```python
from build123d import *

# Parameters (mm, degrees)
CROQUIS1_W                  = 248.76
CROQUIS1_H                  = 195
SALIENTE_EXTRUIR1_DEPTH     = 5
CROQUIS2_W                  = 48
CROQUIS2_H                  = 30
CROQUIS2_W_2                = 30
CORTAR_EXTRUIR1_DEPTH       = 2
CROQUIS3_R                  = 2.375
CORTAR_EXTRUIR2_DEPTH       = 10
CROQUIS4_R                  = 40
SALIENTE_EXTRUIR2_DEPTH     = 206
CROQUIS5_R                  = 12.5
CORTAR_EXTRUIR3_DEPTH       = 10
CROQUIS12_W                 = 12
CROQUIS12_H                 = 30
SALIENTE_EXTRUIR3_DEPTH     = 4
REDONDEO1_R                 = 10
REDONDEO2_R                 = 10
REDONDEO3_R                 = 10
CORTAR_EXTRUIR5_DEPTH       = 262.677217236
CORTAR_EXTRUIR5_DEPTH_BACK  = 262.677217236
CROQUIS13_R                 = 1.625
CORTAR_EXTRUIR7_DEPTH       = 2
CROQUIS16_R                 = 1.75
CORTAR_EXTRUIR9_DEPTH       = 20
CROQUIS17_W                 = 120.38
CROQUIS17_H                 = 213.212791717
CORTAR_EXTRUIR10_DEPTH      = 222
CORTAR_EXTRUIR14_DEPTH      = 165.272498417
CORTAR_EXTRUIR14_DEPTH_BACK = 165.272498417
CROQUIS18_W                 = 124.38
CROQUIS18_H                 = 195


with BuildPart() as part:
    # Croquis1 → Saliente-Extruir1 (new body)
    with BuildSketch(Plane.XY):
        with Locations((7.088293187, 0.26268)):
            Rectangle(CROQUIS1_W, CROQUIS1_H)
    extrude(amount=SALIENTE_EXTRUIR1_DEPTH)

    # Croquis2 → Cortar-Extruir1 (cut)
    with BuildSketch(Plane.XY.offset(5)):
        with Locations((-93.291706813, -82.23732)):
            Rectangle(CROQUIS2_W, CROQUIS2_H)
        with Locations((116.468293187, 82.76268)):
            Rectangle(CROQUIS2_W_2, CROQUIS2_H)
        with Locations((116.468293187, -82.23732)):
            Rectangle(CROQUIS2_W_2, CROQUIS2_H)
        with Locations((-93.291706813, 82.76268)):
            Rectangle(CROQUIS2_W, CROQUIS2_H)
    extrude(amount=-CORTAR_EXTRUIR1_DEPTH, mode=Mode.SUBTRACT)

    # Croquis3 → Cortar-Extruir2 (cut)
    with BuildSketch(Plane.XY.offset(5)):
        with Locations((-93.291706813, 83.76268)):
            Circle(CROQUIS3_R)
        with Locations((-93.291706813, -83.23732)):
            Circle(CROQUIS3_R)
        with Locations((116.468293187, 83.76268)):
            Circle(CROQUIS3_R)
        with Locations((116.468293187, -83.23732)):
            Circle(CROQUIS3_R)
    extrude(amount=-CORTAR_EXTRUIR2_DEPTH, mode=Mode.SUBTRACT)

    # Croquis4 → Saliente-Extruir2 (add)
    with BuildSketch(Plane(origin=(0, 0, 0), x_dir=(-1, 0, 0), z_dir=(0, 0, -1))):
        with Locations(Location((55.101706813, 0.26268, 0), (0, 0, 180))):
            Circle(CROQUIS4_R)
    extrude(amount=SALIENTE_EXTRUIR2_DEPTH)

    # Croquis5 → Cortar-Extruir3 (cut)
    with BuildSketch(Plane(origin=(0, 0, 0), x_dir=(-1, 0, 0), z_dir=(0, 0, -1))):
        with Locations((-76.968293187, 0.26268)):
            Circle(CROQUIS5_R)
    extrude(amount=-CORTAR_EXTRUIR3_DEPTH, mode=Mode.SUBTRACT)

    # Croquis12 → Saliente-Extruir3 (add, symmetric)
    with BuildSketch(Plane(origin=(7.088293187, 0, 0), x_dir=(0, 0, -1), z_dir=(1, 0, 0))):
        with Locations((6, 82.76268)):
            Rectangle(CROQUIS12_W, CROQUIS12_H)
        with Locations((6, -82.23732)):
            Rectangle(CROQUIS12_W, CROQUIS12_H)
    extrude(amount=SALIENTE_EXTRUIR3_DEPTH, both=True)

    # Redondeo1
    redondeo1_edges = [part.edges().sort_by_distance(p)[0] for p in [
        (7.088293187, 67.76268, 0),
        (7.088293187, -67.23732, 0),
    ]]
    fillet(redondeo1_edges, radius=REDONDEO1_R)

    # Redondeo2
    redondeo2_edges = [part.edges().sort_by_distance(p)[0] for p in [
        (7.088293187, 67.76268, -12),
        (7.088293187, -67.23732, -12),
    ]]
    fillet(redondeo2_edges, radius=REDONDEO2_R)

    # Redondeo3
    redondeo3_edges = [part.edges().sort_by_distance(p)[0] for p in [
        (7.088293187, 97.76268, -12),
        (7.088293187, -97.23732, -12),
    ]]
    fillet(redondeo3_edges, radius=REDONDEO3_R)

    # Croquis13 → Cortar-Extruir5 (cut, two sides: drawn at the far end of the back side and taken through both)
    with BuildSketch(Plane(origin=(11.088293187, 0, 0), x_dir=(0, 0, -1), z_dir=(1, 0, 0)).offset(-CORTAR_EXTRUIR5_DEPTH_BACK)):
        with Locations(Location((6, 87.76268, 0), (0, 0, 90))):
            Circle(CROQUIS13_R)
        with Locations(Location((6, 77.76268, 0), (0, 0, 90))):
            Circle(CROQUIS13_R)
        with Locations(Location((6, -77.23732, 0), (0, 0, 90))):
            Circle(CROQUIS13_R)
        with Locations(Location((6, -87.23732, 0), (0, 0, 90))):
            Circle(CROQUIS13_R)
    extrude(amount=CORTAR_EXTRUIR5_DEPTH + CORTAR_EXTRUIR5_DEPTH_BACK, mode=Mode.SUBTRACT)

    # Croquis15 → Cortar-Extruir7 (cut)
    with BuildSketch(Plane.XY.offset(5)):
        Polygon((111.468293187, 67.76268), (131.468293187, 67.76268), (131.468293187, -67.23732), (111.468293187, -67.23732), (111.468293187, -59.48732), (125.218293187, -59.48732), (125.218293187, 60.01268), (111.468293187, 60.01268), align=None)
    extrude(amount=-CORTAR_EXTRUIR7_DEPTH, mode=Mode.SUBTRACT)

    # Croquis16 → Cortar-Extruir9 (cut)
    with BuildSketch(Plane.XY.offset(5)):
        with Locations((-55.101706813, 20.26268)):
            Circle(CROQUIS16_R)
        with Locations((-35.101706813, 0.26268)):
            Circle(CROQUIS16_R)
        with Locations((-55.101706813, -19.73732)):
            Circle(CROQUIS16_R)
        with Locations((-75.101706813, 0.26268)):
            Circle(CROQUIS16_R)
    extrude(amount=-CORTAR_EXTRUIR9_DEPTH, mode=Mode.SUBTRACT)

    # Croquis17 → Cortar-Extruir10 (cut)
    with BuildSketch(Plane.XZ.offset(97.23732)):
        with Locations((-57.101706813, -106.606395859)):
            Rectangle(CROQUIS17_W, CROQUIS17_H)
    extrude(amount=-CORTAR_EXTRUIR10_DEPTH, mode=Mode.SUBTRACT)

    # Croquis18 → Cortar-Extruir14 (cut, two sides: drawn at the far end of the back side and taken through both)
    with BuildSketch(Plane(origin=(0, 0, 0), x_dir=(-1, 0, 0), z_dir=(0, 0, -1)).offset(-CORTAR_EXTRUIR14_DEPTH_BACK)):
        with Locations((-69.278293187, 0.26268)):
            Rectangle(CROQUIS18_W, CROQUIS18_H)
    extrude(amount=CORTAR_EXTRUIR14_DEPTH + CORTAR_EXTRUIR14_DEPTH_BACK, mode=Mode.SUBTRACT)


solid = part.part
```
Build history of the part. All positions in model axes, mm. A direction names the side the tool comes from. Round coordinates to 2 decimals unless told otherwise and drop trailing zeros. Loops run counter-clockwise (first coordinate to the right, second up) from the corner with the lowest first, then second, coordinate; pieces in that order, holes last.
Item 1: Drill centre lines: line 1 along Z through (x, y) = (-69, 85); line 2 along X through (y, z) = (-82, -4.5); line 3 along Z through (x, y) = (-87.5, 72.5). Where is each one in solid material? Low to high.
Item 2: Two-plate mould, pull along Y, no slides. Class faces 1 (the face through (-53.433, -19.212, 2.535)), 2 (the face through (-42, 97.763, 2)), 3 (the face through (-56, 2, 5)): released by +Y, released by -Y, zero draft, split by the parting line, or undercut.
Item 3: Pin check, flat tips, straight feed: P1, Ø3.5, axis at y = 69.5, z = -6, coming from the -X side; P2, Ø4.5, axis at x = -55.1, y = -19.74, coming from the -Z side; P3, Ø0.6, axis at x = -86, z = 4.5, coming from the -Y side. Stop position of each tip, or through.
Item 4: Saw through at C-C (x = -7). List the corners of the cut face in (y, z), then the cut area to 3 significant figures.
Item 5: Saw through at B-B (y = 49). List the corners of the cut face in (x, z).
Item 6: Saw through at A-A (x = -107). List the corners of the cut face in (y, z).
Item 7: Which spindle directions (+Z, -Z, +X, -X, +Y, -Y) get a long thin tool onto all of the face, cutting with end or side? Do faces 4 (the face through (3.088, -81, -6)), 5 (the face through (-93.6, 86.3, 3)), 6 (the face through (5, -81, -12)), 7 (the face through (-94, -79, 3)), 8 (the face through (5.12, 63.17, -1.59)). Say none if no direction does.
Worked answers:
1. line 1: z = 0 to 5
1. line 2: x = 3.09 to 7.09
1. line 3: z = 0 to 3
2. face 1: undercut
2. face 2: released by +Y
2. face 3: zero draft
3. P1: stops at x = 3.09
3. P2: stops at z = 0
3. P3: stops at y = -67.24
4. outline: (-97.24, 0) - (97.76, 0) - (97.76, 5) - (-97.24, 5) - close
4. area: 975 mm2
5. outline: (-117.29, 0) - (7.09, 0) - (7.09, 5) - (-117.29, 5) - close
6. outline: (-97.24, 0) - (97.76, 0) - (97.76, 3) - (67.76, 3) - (67.76, 5) - (-67.24, 5) - (-67.24, 3) - (-97.24, 3) - close
7. face 4: -Z, -X, +Y, -Y
7. face 5: +Z, -X, +Y
7. face 6: -Z, +X, -X, +Y, -Y
7. face 7: +Z, -X, -Y
7. face 8: -Z, +X, -X
